from build123d import *

# Parameters (mm, degrees)
CROQUIS1_W                   = 431.8
CROQUIS1_H                   = 76.2
SALIENTE_EXTRUIR2_DEPTH      = 12.7
CROQUIS3_R                   = 4.826
SALIENTE_EXTRUIR4_DEPTH      = 63.5
CROQUIS4_R                   = 22.479
CORTAR_EXTRUIR3_DEPTH        = 219.71
CROQUIS6_R                   = 22.479
CORTAR_EXTRUIR5_DEPTH        = 180.594
SALIENTE_EXTRUIR5_DEPTH      = 12.7
CROQUIS8_R                   = 22.479
CORTAR_EXTRUIR7_DEPTH        = 46.736
CORTAR_EXTRUIR7_DEPTH_BACK   = 115.062
CROQUIS9_R                   = 22.479
CORTAR_EXTRUIR8_DEPTH        = 153.162
CORTAR_EXTRUIR8_DEPTH_BACK   = 103.886
CROQUIS10_R                  = 4.826
SALIENTE_EXTRUIR6_DEPTH      = 10.414
SALIENTE_EXTRUIR6_DEPTH_BACK = 75.184
CROQUIS12_R                  = 4.826
SALIENTE_EXTRUIR7_DEPTH      = 76.2
SALIENTE_EXTRUIR7_DEPTH_BACK = 13.208


with BuildPart() as part:
    # Croquis1 → Saliente-Extruir2 (new body)
    with BuildSketch(Plane(origin=(0, 0, 0), x_dir=(1, 0, 0), z_dir=(0, 1, 0))):
        with Locations((108.703948782, 38.1)):
            Rectangle(CROQUIS1_W, CROQUIS1_H)
    extrude(amount=SALIENTE_EXTRUIR2_DEPTH)

    # Croquis3 → Saliente-Extruir4 (add)
    with BuildSketch(Plane(origin=(0, 0, 0), x_dir=(1, 0, 0), z_dir=(0, 1, 0))):
        with Locations((-53.918932068, 38.1)):
            Circle(CROQUIS3_R)
        with Locations((51.017757536, 38.1)):
            Circle(CROQUIS3_R)
    extrude(amount=SALIENTE_EXTRUIR4_DEPTH)

    # Croquis4 → Cortar-Extruir3 (cut)
    with BuildSketch(Plane(origin=(0, 0, 0), x_dir=(1, 0, 0), z_dir=(0, 1, 0))):
        with Locations((275.131003884, 35.107884956)):
            Circle(CROQUIS4_R)
    extrude(amount=CORTAR_EXTRUIR3_DEPTH, mode=Mode.SUBTRACT)

    # Croquis6 → Cortar-Extruir5 (cut)
    with BuildSketch(Plane(origin=(0, 0, 0), x_dir=(1, 0, 0), z_dir=(0, 1, 0))):
        with Locations((275.131003884, 35.107884956)):
            Circle(CROQUIS6_R)
    extrude(amount=CORTAR_EXTRUIR5_DEPTH, mode=Mode.SUBTRACT)

    # Croquis7 → Saliente-Extruir5 (add)
    with BuildSketch(Plane(origin=(0, 50.8, 0), x_dir=(1, 0, 0), z_dir=(0, 1, 0))):
        Polygon((-107.196051218, 0), (-107.196051218, 76.439679068), (324.603948782, 76.2), (324.603948782, 0), align=None)
    extrude(amount=SALIENTE_EXTRUIR5_DEPTH)

    # Croquis8 → Cortar-Extruir7 (cut, two sides)
    with BuildSketch(Plane.XZ) as cortar_extruir7_sk:
        with Locations((275.131003884, -35.107884956)):
            Circle(CROQUIS8_R)
    extrude(amount=CORTAR_EXTRUIR7_DEPTH, mode=Mode.SUBTRACT)
    extrude(cortar_extruir7_sk.sketch, amount=-CORTAR_EXTRUIR7_DEPTH_BACK, mode=Mode.SUBTRACT)

    # Croquis9 → Cortar-Extruir8 (cut, two sides)
    with BuildSketch(Plane(origin=(0, 0, 0), x_dir=(1, 0, 0), z_dir=(0, 1, 0))) as cortar_extruir8_sk:
        with Locations((-69.256061559, 35.107884956)):
            Circle(CROQUIS9_R)
    extrude(amount=CORTAR_EXTRUIR8_DEPTH, mode=Mode.SUBTRACT)
    extrude(cortar_extruir8_sk.sketch, amount=-CORTAR_EXTRUIR8_DEPTH_BACK, mode=Mode.SUBTRACT)

    # Croquis10 → Saliente-Extruir6 (add, two sides)
    with BuildSketch(Plane(origin=(0, 63.5, 0), x_dir=(1, 0, 0), z_dir=(0, 1, 0))) as saliente_extruir6_sk:
        with Locations((158.865028896, 34.905026744)):
            Circle(CROQUIS10_R)
    extrude(amount=SALIENTE_EXTRUIR6_DEPTH)
    extrude(saliente_extruir6_sk.sketch, amount=-SALIENTE_EXTRUIR6_DEPTH_BACK)

    # Croquis12 → Saliente-Extruir7 (add, two sides)
    with BuildSketch(Plane(origin=(0, 0, 0), x_dir=(1, 0, 0), z_dir=(0, 1, 0))) as saliente_extruir7_sk:
        with Locations((50.915028896, 34.905026744)):
            Circle(CROQUIS12_R)
    extrude(amount=SALIENTE_EXTRUIR7_DEPTH)
    extrude(saliente_extruir7_sk.sketch, amount=-SALIENTE_EXTRUIR7_DEPTH_BACK)


solid = part.part
Verification items for the finished model (mm, model axes). A direction names the side the tool comes from. Round coordinates to 2 decimals unless told otherwise and drop trailing zeros. Write each loop counter-clockwise with the first axis right and the second up, starting at its lowest first coordinate (ties: lowest second). Pieces come first, ordered by that corner, then holes.
(1) Section check D-D (y = 55). Enter the section's corners in (x, z).
Returned:
outline: (-107.2, -76.44) - (324.6, -76.2) - (324.6, 0) - (-107.2, 0) - close; hole circle Ø44.96 at (-69.26, -35.11); hole circle Ø44.96 at (275.13, -35.11)
(2) Depth check by flat-ended pin: pin 1 Ø23 at (x, z) = (179, -27.5) entering from +Y; pin 2 Ø7.5 at (x, z) = (158.5, -34) entering from -Y; pin 3 Ø10.5 at (x, z) = (157.5, -34) entering from +Y. Enter the tip coordinate at first touch or a pass-through.
Returned:
pin 1: stops at y = 63.5
pin 2: stops at y = -11.68
pin 3: stops at y = 73.91
(3) Mould release check, pull along Y, two halves, no side actions. Record for faces 1 (the flat face through (112, 50.8, -39)), 2 (the cylindrical face through (154.044, -5.76, -35.117)), 3 (the flat face through (51, 76.2, -35)): pulls with the +Y half, pulls with the -Y half, needs draft (parallel to the pull), parting line crosses it, or undercut.
Returned:
face 1: undercut
face 2: needs draft
face 3: pulls with the +Y half
(4) Section check C-C (z = -52). Enter the section's corners in (x, y), plus the area to 3 significant figures.
Returned:
outline: (-107.2, 0) - (-84.09, 0) - (-84.09, 12.7) - (-107.2, 12.7) - close; (-107.2, 50.8) - (-84.09, 50.8) - (-84.09, 63.5) - (-107.2, 63.5) - close; (-54.42, 0) - (260.3, 0) - (260.3, 12.7) - (-54.42, 12.7) - close; (-54.42, 50.8) - (260.3, 50.8) - (260.3, 63.5) - (-54.42, 63.5) - close; (289.96, 0) - (324.6, 0) - (324.6, 12.7) - (289.96, 12.7) - close; (289.96, 50.8) - (324.6, 50.8) - (324.6, 63.5) - (289.96, 63.5) - close
area: 9,460 mm2
(5) Section check A-A (x = -23). Enter the section's corners in (y, z).
Returned:
outline: (0, -76.2) - (12.7, -76.2) - (12.7, 0) - (0, 0) - close; (50.8, -76.39) - (63.5, -76.39) - (63.5, 0) - (50.8, 0) - close
(6) Material ranges on line 1 (Y direction, x = 18, z = -16.5); line 2 (X direction, y = 61.5, z = -17.5); line 3 (X direction, y = 8.5, z = -22.5), recorded low to high.
Returned:
line 1: y = 0 to 12.7, 50.8 to 63.5
line 2: x = -107.2 to -83.23, -55.28 to 261.16, 289.1 to 324.6
line 3: x = -107.2 to -87.87, -50.65 to 256.52, 293.74 to 324.6
(7) Section check B-B (x = -81). Enter the section's corners in (y, z), plus the area to 3 significant figures.
Returned:
outline: (0, -76.2) - (12.7, -76.2) - (12.7, -54.28) - (0, -54.28) - close; (0, -15.94) - (12.7, -15.94) - (12.7, 0) - (0, 0) - close; (50.8, -76.43) - (63.5, -76.43) - (63.5, -54.28) - (50.8, -54.28) - close; (50.8, -15.94) - (63.5, -15.94) - (63.5, 0) - (50.8, 0) - close
area: 965 mm2
(8) Access from +Z, -Z, +X, -X, +Y, -Y to the whole of each face (thin tool, end or side, straight path). Record for faces 4 (the cylindrical face through (50.631, 31.483, -30.087)), 5 (the flat face through (159, -11.684, -35)), 6 (the cylindrical face through (53.509, 69.761, -38.974)), 7 (the cylindrical face through (53.509, -6.512, -38.974)).
Returned:
face 4: none
face 5: +Z, -Z, +X, -Y
face 6: +Y
face 7: -Y
